Design review of the part built by this model. Coordinates are the model's own, in mm. Face numbers are marked on the shaded views. Round coordinates to 2 decimals unless told otherwise and drop trailing zeros. Order: outer loops, then holes, each group sorted by start corner. A loop starts at its lowest first (then second) coordinate and runs counter-clockwise, first axis right, second up.
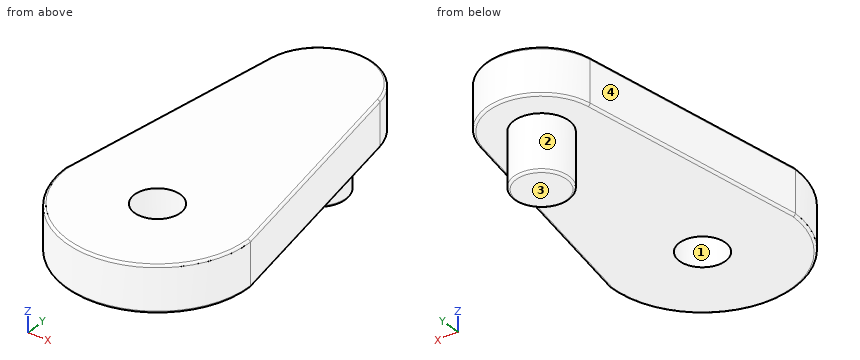
Autodesk Inventor part; units mm, degrees
ref_plane "YZ Plane" through (0, 0, 0) normal (1, 0, 0) x (0, 1, 0)
ref_plane "XZ Plane" through (0, 0, 0) normal (0, 1, 0) x (-1, 0, 0)
ref_plane "XY Plane" through (0, 0, 0) normal (0, 0, 1) x (1, 0, 0)
sketch "Sketch1" plane through (0, 0, 0) normal (0, 0, 1) x (1, 0, 0)
  line L0 (-10, 0) -> (10, 0) construction
  arc A0 (-10, 0) -> (10, 0) centre (0, 0) ccw
  line L1 (-10, 0) -> (-5.9215, 24.9673)
  arc A1 (5.9215, 24.9673) -> (-5.9215, 24.9673) centre (0, 24) ccw
  line L2 (5.9215, 24.9673) -> (10, 0)
  line L3 (0, 0) -> (0, 15.7423) construction
  dimension "d0" = 24
  dimension "d1" = 6
  dimension "d2" = 10
extrude "Extrusion1" add sketch "Sketch1" against normal blind 5
sketch "Sketch2" plane through (0, 0, 0) normal (0, 0, 1) x (1, 0, 0)
  circle A0 centre (0, 24) radius 3
  arc A1 (5.9215, 24.9673) -> (-5.9215, 24.9673) centre (0, 24) ccw
  point P0 (0, 0)
  dimension "d5" = 6
extrude "Extrusion2" add sketch "Sketch2" against normal blind 11
sketch "Sketch3" plane through (0, 0, 0) normal (0, 0, 1) x (1, 0, 0)
  circle A0 centre (0, 0) radius 2.5
  dimension "d14" = 5
extrude "Extrusion3" cut sketch "Sketch3" against normal up to surface (5 mm away)
fillet "Fillet1" radius 0.25 9 edges at (-3, 24, -11) (0, 30, -5) (-7.9608, 12.4836, -5) (7.9608, 12.4836, -5) (0, -10, -5) (0, -10, 0) (0, 30, 0) (-7.9608, 12.4836, 0) (7.9608, 12.4836, 0)
properties part number "201 part 2"
1) Clearance check with flat-ended pins moving along their axes: P1, Ø2, axis at y = 6.5, z = -4, coming from the -X side; P2, Ø5, axis at x = 4.5, z = -1, coming from the -Y side; P3, Ø9.5, axis at x = -3, y = 11.5, coming from the -Z side. State where each tip first meets the part, or that it passes through.
Results:
P1: stops at x = -9.1
P2: stops at y = -9.8
P3: stops at z = -5
2) To check wall thickness, follow line 1 along Y through (x, z) = (0, -1.85); line 2 along Z through (x, y) = (3.25, 25); line 3 along X through (y, z) = (2, -1.25). State the ranges of each line that lie inside material, in increasing order.
Results:
line 1: y = -10 to -2.5, 2.5 to 30
line 2: z = -5 to 0
line 3: x = -9.67 to -1.5, 1.5 to 9.67
3) The part is to be moulded in two halves that separate along Y. For the marked faces 1, 2, 3 and 4, say which applies: released by +Y, released by -Y, zero draft, split by the parting line, or undercut.
Results:
face 1: undercut
face 2: split by the parting line
face 3: zero draft
face 4: released by +Y
4) Take a section at A-A on x = 0. Give the boundary of the cut face in (y, z), plus the area to 3 significant figures.
Results:
outline: (-10, -4.75) arc R0.25 ccw to (-9.75, -5) - (-2.5, -5) - (-2.5, 0) - (-9.75, 0) arc R0.25 ccw to (-10, -0.25) - close; (2.5, -5) - (21, -5) - (21, -10.75) arc R0.25 ccw to (21.25, -11) - (26.75, -11) arc R0.25 ccw to (27, -10.75) - (27, -5) - (29.75, -5) arc R0.25 ccw to (30, -4.75) - (30, -0.25) arc R0.25 ccw to (29.75, 0) - (2.5, 0) - close
area: 211 mm2
5) Take a section at B-B on z = -5.75. Give the boundary of the cut face in (x, y).
Results:
outline: circle Ø6 at (0, 24)
